Here's how the part is built. I have some questions about the finished solid (model axes, mm). Coordinates: 2 decimals unless noted, no trailing zeros. Write each loop counter-clockwise with the first axis right and the second up, starting at its lowest first coordinate (ties: lowest second). Pieces come first, ordered by that corner, then holes. Notation, with made-up numbers: (71.25, 86.5) -> (122.25, 86.5) arc R24 ccw to (122.25, 117.5) -> close; hole circle Ø9 at (9, 68.5). An arc over 180 degrees is marked (long way). Put each result on its own line as item: value.
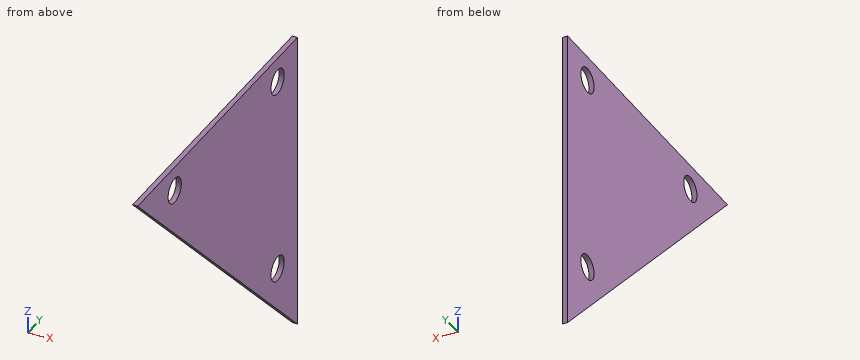
```python
from build123d import *

# Parameters (mm, degrees)
BOSS_EXTRUDE1_DEPTH                            = 2.54
CSK_FOR_M6_FLAT_HEAD_MACHINE_SCREW1_AT_2_COUNT = 2
CSK_FOR_M6_FLAT_HEAD_MACHINE_SCREW1_AT_2_PITCH = 99.31634163
CSK_FOR_M6_FLAT_HEAD_MACHINE_SCREW1_AT_3_COUNT = 2
CSK_FOR_M6_FLAT_HEAD_MACHINE_SCREW1_AT_3_PITCH = 98.119759201


with BuildPart() as part:
    # Sketch1 → Boss-Extrude1 (new body)
    with BuildSketch(Plane(origin=(0, 0, 0), x_dir=(0, 0, -1), z_dir=(1, 0, 0))):
        Polygon((112.940672783, 23.924159021), (-39.459327217, -128.475840979), (-39.459327217, 23.924159021), align=None)
    extrude(amount=BOSS_EXTRUDE1_DEPTH)

    # Sketch3 → CSK for M6 Flat Head Machine Screw1 (revolve, cut)
    with BuildSketch(Plane(origin=(2.54, 5.007497158, 27.039858725), x_dir=(0, 0, -1), z_dir=(0, 1, 0))):
        Polygon((0, 0), (0, 2.54), (3.3, 2.54), (3.3, 28.4), (6.3, 25.4), (6.3, 0), align=None)
    csk_for_m6_flat_head_machine_screw1 = revolve(axis=Axis((8.89, 5.007497158, 27.039858725), (-1, 0, 0)), mode=Mode.SUBTRACT)

    # CSK for M6 Flat Head Machine Screw1 at 2: CSK for M6 Flat Head Machine Screw1 ×2
    with Locations(*[(0, 0, -i * CSK_FOR_M6_FLAT_HEAD_MACHINE_SCREW1_AT_2_PITCH) for i in range(1, CSK_FOR_M6_FLAT_HEAD_MACHINE_SCREW1_AT_2_COUNT)]):
        add(csk_for_m6_flat_head_machine_screw1, mode=Mode.SUBTRACT)

    # CSK for M6 Flat Head Machine Screw1 at 3: CSK for M6 Flat Head Machine Screw1 ×2
    with Locations(*[(0, -i * CSK_FOR_M6_FLAT_HEAD_MACHINE_SCREW1_AT_3_PITCH, 0) for i in range(1, CSK_FOR_M6_FLAT_HEAD_MACHINE_SCREW1_AT_3_COUNT)]):
        add(csk_for_m6_flat_head_machine_screw1, mode=Mode.SUBTRACT)


solid = part.part
```
Item 1: Imagine slicing it at A-A on x = 0.75. Write out the boundary of the cut face in (y, z).
Output:
outline: (-128.48, 39.46) -> (23.92, -112.94) -> (23.92, 39.46) -> close; hole circle Ø12.6 at (-93.11, 27.04); hole circle Ø12.6 at (5.01, -72.28); hole circle Ø12.6 at (5.01, 27.04)
Item 2: Imagine slicing it at C-C on z = -23. Write out the boundary of the cut face in (x, y), then the cut area to 3 significant figures.
Output:
outline: (0, -66.02) -> (2.54, -66.02) -> (2.54, 23.92) -> (0, 23.92) -> close
area: 228 mm²
Item 3: Please list where these lines run through material, in increasing order: line 1 along Z through (x, y) = (1.8, 5); line 2 along Y through (x, z) = (1.5, -69.5); line 3 along Z through (x, y) = (0.6, -95). Write a range as from..to.
Output:
line 1: z = -94.02..-78.58, -65.98..20.74, 33.34..39.46
line 2: y = -19.52..-0.65, 10.66..23.92
line 3: z = 5.98..21.03, 33.05..39.46
Item 4: Imagine slicing it at B-B on y = -11. Write out the boundary of the cut face in (x, z).
Output:
outline: (0, -78.02) -> (2.54, -78.02) -> (2.54, 39.46) -> (0, 39.46) -> close
